```python
from build123d import *

# Parameters (mm, degrees)
F2_SIZE  = 2
F3_R     = 2.5
F4_R     = 6.25
F5_DEPTH = 14.2


with BuildPart() as f1:
    # F0 (on Front) → F1 (revolve)
    with BuildSketch(Plane.XZ):
        Polygon((-20, 58.4), (-20, 14.2), (-45, 14.2), (-45, 0), (-15, 0), (-15, 64.4), (-19, 64.4), (-19, 88.4), (-25, 88.4), (-25, 58.4), align=None)
    revolve(axis=Axis((0, 0, 34.592547), (0, 0, 1)))

    # F2
    f2_edges = [f1.edges().sort_by_distance(p)[0] for p in [
        (15, 0, 0),
        (19, 0, 88.4),
        (19, 0, 64.4),
    ]]
    chamfer(f2_edges, length=F2_SIZE)

    # F3
    f3_edges = [f1.edges().sort_by_distance(p)[0] for p in [
        (20, 0, 14.2),
        (20, 0, 58.4),
        (45, 0, 14.2),
    ]]
    fillet(f3_edges, radius=F3_R)

    # F4 (on face) → F5 (cut, through all)
    with BuildSketch(Plane.XY.offset(14.2)):
        with Locations((0, 34)):
            Circle(F4_R)
        with Locations((-34, 0)):
            Circle(F4_R)
        with Locations((0, -34)):
            Circle(F4_R)
        with Locations((34, 0)):
            Circle(F4_R)
    extrude(amount=-F5_DEPTH, mode=Mode.SUBTRACT)


solid = f1.part
```
The model under review builds one solid part; all positions refer to its coordinate system, in mm. A direction names the side the tool comes from. Coordinates: 2 decimals unless noted, no trailing zeros. Write each loop counter-clockwise with the first axis right and the second up, starting at its lowest first coordinate (ties: lowest second). Pieces come first, ordered by that corner, then holes. Notation, with made-up numbers: (8.5, 89.5) - (19.5, 89.5) arc R29 cw to (19.5, 113.5) - close; hole circle Ø10 at (60.5, 29). An arc over 180 degrees is marked (long way). Answer in a Markdown table with one row per item. Add a question column.
Q1. To check wall thickness, follow line 1 along Y through (x, z) = (0, 9); line 2 along X through (y, z) = (0, 80.75). State the ranges of each line that lie inside material, in increasing order. Write a range as from..to.
Q2. Consider section C-C on x = -1.5. Give the number of separate pieces and of enclosed holes in the cut face, then the cut area to 3 significant figures.
Q3. Clearance check with flat-ended pins moving along their axes: pin 1 (7.5 mm diameter, centred on x = 0, y = -34, fed in from -Z); pin 2 (1 mm diameter, centred on x = -8, z = 68, fed in from -Y); pin 3 (4 mm diameter, centred on y = -20.5, z = 13.5, fed in from -X); pin 4 (5 mm diameter, centred on y = 6, z = 50, fed in from -X). State where each tip first meets the part, or that it passes through.
Q4. Consider section B-B on z = 6. Give the boundary of the cut face in (x, y), then the cut area to 3 significant figures.
Q5. For faces 1 (the face through (4.336, 19.524, 36.026)), 2 (the face through (-40.244, 0.275, 7.199)), 3 (the face through (6, 14, 64.4)), list the 3-axis set-ups (+Z, -Z, +X, -X, +Y, -Y) from which the entire face can be reached by the end or side of a thin tool; tool diameter is ignored.
Q6. Draft analysis for pull direction X (two halves, no side actions). For faces 4 (the face through (-5.7, -20.5, 88.4)), 5 (the face through (29.04, -3.8, 7.2)), 6 (the face through (-23.846, -7.509, 73.19)), state which applies: +X half, -X half, draft (parallel to the pull), parting line (faces both ways), or undercut.
Q7. Consider section A-A on z = 47. Give the boundary of the cut face in (x, y), then the cut area to 3 significant figures.
Answers below:
| question | item | result |
|---|---|---|
| 1 | line 1 | -45..-40.25, -27.75..-15, 15..27.75, 40.25..45 |
| 1 | line 2 | -25..-19, 19..25 |
| 2 | separate pieces | 4 |
| 2 | enclosed holes | 0 |
| 2 | area | 1,360 mm² |
| 3 | pin 1 | through |
| 3 | pin 2 | y = -23.85 |
| 3 | pin 3 | x = -40.76 |
| 3 | pin 4 | x = -19.69 |
| 4 | outline | circle Ø90 at (0, 0); hole circle Ø12.5 at (-34, 0); hole circle Ø30 at (0, 0); hole circle Ø12.5 at (0, -34); hole circle Ø12.5 at (0, 34); hole circle Ø12.5 at (34, 0) |
| 4 | area | 5,160 mm² |
| 5 | face 1 | none |
| 5 | face 2 | +Z, -Z |
| 5 | face 3 | +Z |
| 6 | face 4 | draft |
| 6 | face 5 | undercut |
| 6 | face 6 | parting line |
| 7 | outline | circle Ø40 at (0, 0); hole circle Ø30 at (0, 0) |
| 7 | area | 550 mm² |
